from build123d import *

# Parameters (mm, degrees)
SKETCH_1_W          = 60
SKETCH_1_H          = 120
SKETCH_1_R          = 1.6
SKETCH_1_R_2        = 2.15
EXTRUDE_3_DEPTH     = 6
SKETCH_9_R          = 1.6
CUT_EXTRUDE_1_DEPTH = 6
FILLET_1_R          = 10
SKETCH_11_R         = 20
SKETCH_11_R_2       = 1.6
CUT_EXTRUDE_2_DEPTH = 6
SKETCH_21_R         = 1.6
CUT_EXTRUDE_7_DEPTH = 10


with BuildPart() as part:
    # 草图1 → 凸台-拉伸3 (new body)
    with BuildSketch(Plane.XY):
        Rectangle(SKETCH_1_W, SKETCH_1_H)
        with Locations((0, 50.5)):
            Circle(SKETCH_1_R, mode=Mode.SUBTRACT)
        with Locations((20, -50)):
            Circle(SKETCH_1_R_2, mode=Mode.SUBTRACT)
        with Locations((-20, -50)):
            Circle(SKETCH_1_R_2, mode=Mode.SUBTRACT)
        with Locations((13.423393759, 42.75)):
            Circle(SKETCH_1_R, mode=Mode.SUBTRACT)
        with Locations((13.423393759, 27.25)):
            Circle(SKETCH_1_R, mode=Mode.SUBTRACT)
        with Locations((0, 19.5)):
            Circle(SKETCH_1_R, mode=Mode.SUBTRACT)
        with Locations((-13.423393759, 27.25)):
            Circle(SKETCH_1_R, mode=Mode.SUBTRACT)
        with Locations((-13.423393759, 42.75)):
            Circle(SKETCH_1_R, mode=Mode.SUBTRACT)
        with BuildLine():
            Line((6, 42), (6, 28))
            ThreePointArc((6, 28), (0, 22), (-6, 28))
            Line((-6, 28), (-6, 42))
            ThreePointArc((-6, 42), (0, 48), (6, 42))
        make_face(mode=Mode.SUBTRACT)
    extrude(amount=EXTRUDE_3_DEPTH)

    # 草图9 → 切除-拉伸1 (cut)
    with BuildSketch(Plane.XY.offset(6)):
        with Locations((20.1, -22)):
            Circle(SKETCH_9_R)
        with Locations((20.1, -2)):
            Circle(SKETCH_9_R)
        with Locations((20.1, -12)):
            Circle(SKETCH_9_R)
        with Locations((-20.1, -2)):
            Circle(SKETCH_9_R)
        with Locations((-20.1, -12)):
            Circle(SKETCH_9_R)
        with Locations((-20.1, -22)):
            Circle(SKETCH_9_R)
    extrude(amount=-CUT_EXTRUDE_1_DEPTH, mode=Mode.SUBTRACT)

    # 圆角1
    fillet_1_edges = [part.edges().sort_by_distance(p)[0] for p in [
        (30, -60, 3),
        (-30, -60, 3),
        (-30, 60, 3),
        (30, 60, 3),
    ]]
    fillet(fillet_1_edges, radius=FILLET_1_R)

    # 草图11 → 切除-拉伸2 (cut)
    with BuildSketch(Plane(origin=(0, 0, 0), x_dir=(-1, 0, 0), z_dir=(0, 0, -1))):
        with Locations((0, 35)):
            Circle(SKETCH_11_R)
        with Locations((-13.423393759, 27.25)):
            Circle(SKETCH_11_R_2, mode=Mode.SUBTRACT)
        with Locations((13.423393759, 27.25)):
            Circle(SKETCH_11_R_2, mode=Mode.SUBTRACT)
        with Locations((13.423393759, 42.75)):
            Circle(SKETCH_11_R_2, mode=Mode.SUBTRACT)
        with Locations((0, 19.5)):
            Circle(SKETCH_11_R_2, mode=Mode.SUBTRACT)
        with Locations((0, 50.5)):
            Circle(SKETCH_11_R_2, mode=Mode.SUBTRACT)
        with Locations((-13.423393759, 42.75)):
            Circle(SKETCH_11_R_2, mode=Mode.SUBTRACT)
        with BuildLine():
            ThreePointArc((-6, 42), (0, 48), (6, 42))
            Line((6, 42), (6, 28))
            ThreePointArc((6, 28), (0, 22), (-6, 28))
            Line((-6, 28), (-6, 42))
        make_face(mode=Mode.SUBTRACT)
    extrude(amount=-CUT_EXTRUDE_2_DEPTH, mode=Mode.SUBTRACT)

    # 草图21 → 切除-拉伸7 (cut)
    with BuildSketch(Plane(origin=(0, 0, 0), x_dir=(-1, 0, 0), z_dir=(0, 0, -1))):
        with Locations((-20, 50)):
            Circle(SKETCH_21_R)
        with Locations(Location((20, 50, 0), (0, 0, 180))):
            Circle(SKETCH_21_R)
        with Locations((25, 10)):
            Circle(SKETCH_21_R)
        with Locations(Location((-25, 10, 0), (0, 0, 180))):
            Circle(SKETCH_21_R)
    extrude(amount=-CUT_EXTRUDE_7_DEPTH, mode=Mode.SUBTRACT)


solid = part.part
Model file for the job. Use its own axes, mm. Round coordinates to 2 decimals unless told otherwise and drop trailing zeros. Loops run counter-clockwise (first coordinate to the right, second up) from the corner with the lowest first, then second, coordinate; pieces in that order, holes last.
1. Band-saw the part on A-A, the plane y = -2. List the corners of the cut face in (x, z), and give its area (3 significant figures).
Check values:
outline: (-30, 0) - (-21.7, 0) - (-21.7, 6) - (-30, 6) - close; (-18.5, 0) - (18.5, 0) - (18.5, 6) - (-18.5, 6) - close; (21.7, 0) - (30, 0) - (30, 6) - (21.7, 6) - close
area: 322 mm2
2. Band-saw the part on D-D, the plane y = 41.5. List the corners of the cut face in (x, z).
Check values:
outline: (-30, 0) - (-18.91, 0) - (-18.91, 6) - (-30, 6) - close; (18.91, 0) - (30, 0) - (30, 6) - (18.91, 6) - close
3. Mould opens along X. For faces 1 (the cylindrical face through (-18.574, -1.519, 3.042)), 2 (the flat face through (0, 1, 6)), 3 (the cylindrical face through (26.99, -57.15, 3.04)) say: +X half, -X half, draft (parallel to the pull), parting line (faces both ways), or undercut.
Check values:
face 1: undercut
face 2: draft
face 3: +X half
4. Wall check: probe 1 along Y at (x, z) = (-20.1, 1.5); probe 2 along Y at (x, z) = (0, 1.85); probe 3 along X at (y, z) = (26, 3.5). Give the ranges that are in metal, low to high.
Check values:
probe 1: y = -60 to -52.15, -47.85 to -23.6, -20.4 to -13.6, -10.4 to -3.6, -0.4 to 48.4, 51.6 to 60
probe 2: y = -60 to 15, 55 to 60
probe 3: x = -30 to -17.86, 17.86 to 30
5. Band-saw the part on C-C, the plane x = 13.5. List the corners of the cut face in (y, z), and give its area (3 significant figures).
Check values:
outline: (-60, 0) - (20.24, 0) - (20.24, 6) - (-60, 6) - close; (49.76, 0) - (60, 0) - (60, 6) - (49.76, 6) - close
area: 543 mm2
6. Band-saw the part on B-B, the plane z = 2.25. Count the separate pieces of the cut face and the enclosed holes in it, and give its area (3 significant figures).
Check values:
separate pieces: 1
enclosed holes: 13
area: 5,750 mm2
7. Drop a flat-ended pin along its axis: P1, Ø1.9, axis at x = -20.1, y = -12, coming from the -Z side (3 decimals). Give the stop position or say it passes through.
Check values:
P1: passes through
